Can you work these out from the model? Positions are in its coordinate system, mm. Round coordinates to 2 decimals unless told otherwise and drop trailing zeros. Write each loop counter-clockwise with the first axis right and the second up, starting at its lowest first coordinate (ties: lowest second). Pieces come first, ordered by that corner, then holes. Notation, with made-up numbers: M -22.75,14.5 L -6.75,14.5 A8 ccw -6.75,27.5 Z; hole C 4.25,66 d4. An arc over 180 degrees is marked long. Use one line per item in the form item = value. Start each with the question number.
```python
from build123d import *

# Parameters (mm, degrees)
BOSS_EXTRUDE1_DEPTH     = 21.9
CUT_EXTRUDE1_DEPTH      = 38.070945496
CUT_EXTRUDE1_DEPTH_BACK = 38.070945496
SKETCH2_R               = 2.75


with BuildPart() as part:
    # Sketch1 → Boss-Extrude1 (new body)
    with BuildSketch(Plane(origin=(0, 0, 0), x_dir=(1, 0, 0), z_dir=(0, 1, 0))):
        with BuildLine():
            Line((-14.442201826, 20.913137233), (-20.913137233, 14.442201826))
            ThreePointArc((-20.913137233, 14.442201826), (-21.088441372, 14.179840641), (-21.15, 13.870364522))
            Line((-21.15, 13.870364522), (-21.15, -13.870364522))
            ThreePointArc((-21.15, -13.870364522), (-21.088441372, -14.179840641), (-20.913137233, -14.442201826))
            Line((-20.913137233, -14.442201826), (-14.442201826, -20.913137233))
            ThreePointArc((-14.442201826, -20.913137233), (-14.179840641, -21.088441372), (-13.870364522, -21.15))
            Line((-13.870364522, -21.15), (13.870364522, -21.15))
            ThreePointArc((13.870364522, -21.15), (14.179840641, -21.088441372), (14.442201826, -20.913137233))
            Line((14.442201826, -20.913137233), (20.913137233, -14.442201826))
            ThreePointArc((20.913137233, -14.442201826), (21.088441372, -14.179840641), (21.15, -13.870364522))
            Line((21.15, -13.870364522), (21.15, 13.870364522))
            ThreePointArc((21.15, 13.870364522), (21.088441372, 14.179840641), (20.913137233, 14.442201826))
            Line((20.913137233, 14.442201826), (14.442201826, 20.913137233))
            ThreePointArc((14.442201826, 20.913137233), (14.179840641, 21.088441372), (13.870364522, 21.15))
            Line((13.870364522, 21.15), (-13.870364522, 21.15))
            ThreePointArc((-13.870364522, 21.15), (-14.179840641, 21.088441372), (-14.442201826, 20.913137233))
        make_face()
    extrude(amount=BOSS_EXTRUDE1_DEPTH)

    # Sketch2 → Cut-Extrude1 (cut, two sides: drawn at the far end of the back side and taken through both)
    with BuildSketch(Plane(origin=(0, 21.9, 0), x_dir=(1, 0, 0), z_dir=(0, 1, 0)).offset(-CUT_EXTRUDE1_DEPTH_BACK)):
        with Locations(Location((0, 0, 0), (0, 0, 270))):
            Circle(SKETCH2_R)
    extrude(amount=CUT_EXTRUDE1_DEPTH + CUT_EXTRUDE1_DEPTH_BACK, mode=Mode.SUBTRACT)


solid = part.part
```
1. Please list where these lines run through material, in increasing order: line 1 along X through (y, z) = (7.75, 0); line 2 along X through (y, z) = (17.5, 2).
2. Will this pin go through, and if not, where does the flat tip stop? pin 1 (6 mm diameter, centred on y = 14.5, z = -15.5, fed in from -X).
3. If we section it at C-C (x = 0): List the corners of the cut face in (y, z) for me.
4. If we mould it in two halves opening along X, with no side actions, what happens to faces 1 (the face through (-5, 21.9, 0)), 2 (the face through (-2.685, 10.797, -0.596)), 3 (the face through (-17.723, 10.797, 17.632))? For each: pulls with the +X half, pulls with the -X half, needs draft (parallel to the pull), parting line crosses it, or undercut.
5. If we section it at D-D (z = -18): List the corners of the cut face in (x, y) for me, and give its area (3 significant figures).
6. If we section it at B-B (y = 17.25): List the corners of the cut face in (x, z) for me.
7. If we section it at A-A (z = 0): List the corners of the cut face in (x, y) for me.
Model answer:
q1.line_1 = -21.15 to -2.75, 2.75 to 21.15
q1.line_2 = -21.15 to -1.89, 1.89 to 21.15
q2.pin_1 = -21.15
q3.outline = M 0,-21.15 L 21.9,-21.15 L 21.9,-2.75 L 0,-2.75 Z; M 0,2.75 L 21.9,2.75 L 21.9,21.15 L 0,21.15 Z
q4.face_1 = needs draft
q4.face_2 = undercut
q4.face_3 = pulls with the -X half
q5.outline = M -17.36,0 L 17.36,0 L 17.36,21.9 L -17.36,21.9 Z
q5.area = 760 mm2
q6.outline = M -21.15,-13.87 A0.81 ccw -20.91,-14.44 L -14.44,-20.91 A0.81 ccw -13.87,-21.15 L 13.87,-21.15 A0.81 ccw 14.44,-20.91 L 20.91,-14.44 A0.81 ccw 21.15,-13.87 L 21.15,13.87 A0.81 ccw 20.91,14.44 L 14.44,20.91 A0.81 ccw 13.87,21.15 L -13.87,21.15 A0.81 ccw -14.44,20.91 L -20.91,14.44 A0.81 ccw -21.15,13.87 Z; hole C 0,0 d5.5
q7.outline = M -21.15,0 L -2.75,0 L -2.75,21.9 L -21.15,21.9 Z; M 2.75,0 L 21.15,0 L 21.15,21.9 L 2.75,21.9 Z
